Geometry: final body of the model. Coordinates: model frame, mm. Face numbers are marked on the shaded views. A direction names the side the tool comes from. Give positions to 0.01 mm unless a question says otherwise; leave off trailing zeros. Loops run counter-clockwise (first coordinate to the right, second up) from the corner with the lowest first, then second, coordinate; pieces in that order, holes last. Notation, with made-up numbers: (16.25, -28.75) -> (27.25, -28.75) arc R12 ccw to (27.25, -23.75) -> close; hole circle Ø9 at (52.5, 29.25). An arc over 180 degrees is marked (long way). One line per question, with ' | ' between items. Start each with the question number.
Item 1: Mould query, pull axis X, two halves, no side actions, for the marked faces 3, 4, 5 and 6. Classes: released by +X, released by -X, zero draft, split by the parting line, or undercut.
Item 2: Section B-B on x = -5. Return loops of the section in (y, z).
Item 3: Section A-A on y = 4. Return loops of the section in (x, z), then the cut area to 4 significant figures.
Item 4: Section D-D on x = -47. Return loops of the section in (y, z).
Item 5: Set-up query: the marked faces 1 and 2. Return all of +Z, -Z, +X, -X, +Y, -Y with unobstructed straight access to the full face (end or side cutting, diameter ignored); none if empty.
Item 6: Pin query (flat end, axial travel): P1, Ø5, axis at x = -5.5, z = 49, coming from the +Y side; P2, Ø1.3, axis at x = -55, z = 53, coming from the +Y side; P3, Ø7, axis at x = -63, z = 18, coming from the +Y side. Return the tip coordinate at first contact, or that it passes through.
Item 7: Section C-C on z = 8. Return loops of the section in (x, y).
Item 8: Material intervals for line 1 along X through (y, z) = (17, 6); line 2 along Z through (x, y) = (-48, 25); line 3 along X through (y, z) = (29.5, 53), sorted ascending. Write a range as [from, to].
from build123d import *

# Parameters (mm, degrees)
SKETCH1_W           = 75.2
SKETCH1_H           = 62
SKETCH1_W_2         = 54
SKETCH1_H_2         = 56
SKETCH1_R           = 3
SKETCH1_W_3         = 1.2
SKETCH1_W_4         = 14
BOSS_EXTRUDE1_DEPTH = 3
BOSS_EXTRUDE2_START = 3
SKETCH1_3_R         = 3
BOSS_EXTRUDE2_DEPTH = 3
BOSS_EXTRUDE3_START = 3
SKETCH1_4_W         = 75.2
SKETCH1_4_H         = 62
SKETCH1_4_W_2       = 1.2
SKETCH1_4_H_2       = 56
BOSS_EXTRUDE3_DEPTH = 33
CUT_EXTRUDE1_REACH  = 103.749
SKETCH2_W           = 9
SKETCH2_H           = 4
CUT_EXTRUDE2_REACH  = 92.356
SKETCH3_W           = 4
SKETCH3_H           = 12
CUT_EXTRUDE3_REACH  = 103.749
SKETCH4_W           = 20
SKETCH4_H           = 16


with BuildPart() as part:
    # Sketch1 → Boss-Extrude1 (new body)
    with BuildSketch(Plane(origin=(0, 0, 0), x_dir=(1, 0, 0), z_dir=(0, 1, 0))):
        with Locations((-34.6, -28)):
            Rectangle(SKETCH1_W, SKETCH1_H)
        Polygon((-55.2, -56), (-54, -56), (0, -56), (0, 0), (-54, 0), (-55.2, 0), (-69.2, 0), (-69.2, -56), align=None, mode=Mode.SUBTRACT)
        with Locations((-27, -28)):
            Rectangle(SKETCH1_W_2, SKETCH1_H_2)
        with Locations((-47, -50)):
            Circle(SKETCH1_R, mode=Mode.SUBTRACT)
        with Locations((-5, -50)):
            Circle(SKETCH1_R, mode=Mode.SUBTRACT)
        with Locations((-5, -8)):
            Circle(SKETCH1_R, mode=Mode.SUBTRACT)
        with Locations((-47, -8)):
            Circle(SKETCH1_R, mode=Mode.SUBTRACT)
        with Locations((-47, -50)):
            Circle(SKETCH1_R)
        with Locations((-5, -50)):
            Circle(SKETCH1_R)
        with Locations((-5, -8)):
            Circle(SKETCH1_R)
        with Locations((-47, -8)):
            Circle(SKETCH1_R)
        with Locations((-54.6, -28)):
            Rectangle(SKETCH1_W_3, SKETCH1_H_2)
        with Locations((-62.2, -28)):
            Rectangle(SKETCH1_W_4, SKETCH1_H_2)
    extrude(amount=BOSS_EXTRUDE1_DEPTH)

    # Sketch1<3> → Boss-Extrude2 (add)
    with BuildSketch(Plane(origin=(0, 0, 0), x_dir=(1, 0, 0), z_dir=(0, 1, 0)).offset(BOSS_EXTRUDE2_START)):
        with Locations(Location((-47, -50, 0), (0, 0, 270))):
            Circle(SKETCH1_3_R)
        with Locations(Location((-5, -50, 0), (0, 0, 270))):
            Circle(SKETCH1_3_R)
        with Locations(Location((-5, -8, 0), (0, 0, 270))):
            Circle(SKETCH1_3_R)
        with Locations(Location((-47, -8, 0), (0, 0, 270))):
            Circle(SKETCH1_3_R)
    extrude(amount=BOSS_EXTRUDE2_DEPTH)

    # Sketch1<4> → Boss-Extrude3 (add)
    with BuildSketch(Plane(origin=(0, 0, 0), x_dir=(1, 0, 0), z_dir=(0, 1, 0)).offset(BOSS_EXTRUDE3_START)):
        with Locations((-34.6, -28)):
            Rectangle(SKETCH1_4_W, SKETCH1_4_H)
        Polygon((-55.2, -56), (-54, -56), (0, -56), (0, 0), (-54, 0), (-55.2, 0), (-69.2, 0), (-69.2, -56), align=None, mode=Mode.SUBTRACT)
        with Locations((-54.6, -28)):
            Rectangle(SKETCH1_4_W_2, SKETCH1_4_H_2)
    extrude(amount=BOSS_EXTRUDE3_DEPTH)

    # Sketch2 → Cut-Extrude1 (cut, up to next)
    with BuildSketch(Plane.XY.offset(59), mode=Mode.PRIVATE) as cut_extrude1_sk1:
        with Locations((-24.5, 9.5)):
            Rectangle(SKETCH2_W, SKETCH2_H)
    cut_extrude1_tool1 = extrude(cut_extrude1_sk1.sketch, amount=-CUT_EXTRUDE1_REACH, mode=Mode.PRIVATE) & part.part
    add(cut_extrude1_tool1.solids().sort_by_distance((-24.5, 9.5, 59))[0], mode=Mode.SUBTRACT)

    # Sketch3 → Cut-Extrude2 (cut, up to next)
    with BuildSketch(Plane.ZY.offset(55.2), mode=Mode.PRIVATE) as cut_extrude2_sk1:
        with Locations((54, 30)):
            Rectangle(SKETCH3_W, SKETCH3_H)
    cut_extrude2_tool1 = extrude(cut_extrude2_sk1.sketch, amount=-CUT_EXTRUDE2_REACH, mode=Mode.PRIVATE) & part.part
    add(cut_extrude2_tool1.solids().sort_by_distance((-55.2, 30, 54))[0], mode=Mode.SUBTRACT)

    # Sketch4 → Cut-Extrude3 (cut, up to next)
    with BuildSketch(Plane(origin=(0, 0, -3), x_dir=(-1, 0, 0), z_dir=(0, 0, -1)), mode=Mode.PRIVATE) as cut_extrude3_sk1:
        with Locations((12, 25)):
            Rectangle(SKETCH4_W, SKETCH4_H)
    cut_extrude3_tool1 = extrude(cut_extrude3_sk1.sketch, amount=-CUT_EXTRUDE3_REACH, mode=Mode.PRIVATE) & part.part
    add(cut_extrude3_tool1.solids().sort_by_distance((-12, 25, -3))[0], mode=Mode.SUBTRACT)


solid = part.part
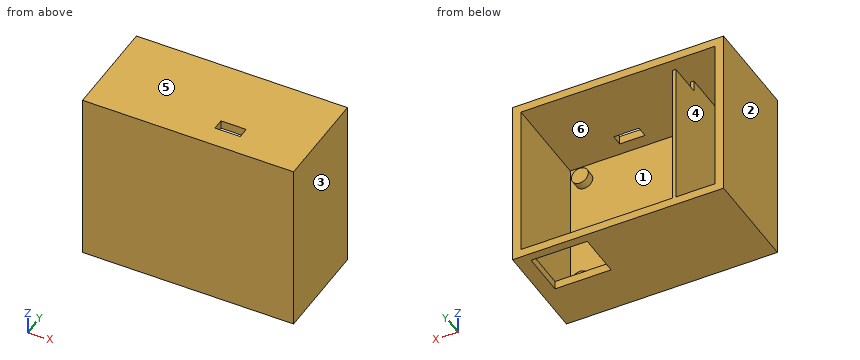
Result sheet:
1) face 3: released by +X | face 4: undercut | face 5: zero draft | face 6: undercut
2) outline: (0, -3) -> (17, -3) -> (17, 0) -> (3, 0) -> (3, 5) -> (6, 5) -> (6, 11) -> (3, 11) -> (3, 47) -> (6, 47) -> (6, 53) -> (3, 53) -> (3, 56) -> (36, 56) -> (36, 59) -> (0, 59) -> close; (33, -3) -> (36, -3) -> (36, 0) -> (33, 0) -> close
3) outline: (-72.2, -3) -> (3, -3) -> (3, 59) -> (-72.2, 59) -> close; circle Ø6 at (-47, 8); circle Ø6 at (-47, 50); circle Ø6 at (-5, 8); circle Ø6 at (-5, 50); hole (-69.2, 0) -> (-55.2, 0) -> (-55.2, 56) -> (-69.2, 56) -> close; hole (-54, 0) -> (0, 0) -> (0, 56) -> (-54, 56) -> close | area: 967.5 mm²
4) outline: (0, -3) -> (36, -3) -> (36, 0) -> (3, 0) -> (3, 5) -> (6, 5) -> (6, 11) -> (3, 11) -> (3, 47) -> (6, 47) -> (6, 53) -> (3, 53) -> (3, 56) -> (36, 56) -> (36, 59) -> (0, 59) -> close
5) face 1: +Y | face 2: +Z, -Z, -X, +Y, -Y
6) P1: stops at y = 6 | P2: stops at y = 24 | P3: stops at y = 3
7) outline: (-72.2, 0) -> (3, 0) -> (3, 36) -> (0, 36) -> (0, 3) -> (-2, 3) -> (-2, 6) -> (-8, 6) -> (-8, 3) -> (-44, 3) -> (-44, 6) -> (-50, 6) -> (-50, 3) -> (-54, 3) -> (-54, 36) -> (-55.2, 36) -> (-55.2, 3) -> (-69.2, 3) -> (-69.2, 36) -> (-72.2, 36) -> close
8) line 1: x = [-72.2, -69.2], [-55.2, -54], [0, 3] | line 2: z = [-3, 0], [56, 59] | line 3: x = [-72.2, -69.2], [0, 3]
